Can you work these out from the model? Positions are in its coordinate system, mm. A direction names the side the tool comes from. Give positions to 0.01 mm unless a question says otherwise; leave off trailing zeros. Loops run counter-clockwise (first coordinate to the right, second up) from the corner with the lowest first, then second, coordinate; pieces in that order, holes last. Notation, with made-up numbers: (56.25, -17.5) -> (79.25, -17.5) arc R22 cw to (79.25, 13.5) -> close; hole circle Ø8 at (41.25, -32). An arc over 180 degrees is marked (long way). Return JSON: item names as keys, results as strings. Group by question number.
Q1. Suppose I cut it at A-A, the plane y = 155. Please give me the cut outline in (x, z) (1 decimal).
Q2. Thinking about a two-plate mould opening in X: for faces 1 (the flat face through (1, 47.625, 181)), 2 (the flat face through (-74.612, 143, 182)), 3 (the flat face through (-1, 143, 188.912)), which applies, pulls with the +X half, pulls with the -X half, needs draft (parallel to the pull), parting line crosses it, or undercut?
Q3. Will these pins go through, and if not, where does the flat tip stop? pin 1 (4 mm diameter, centred on x = 42, y = 159.5, fed in from -Z) (3 decimals); pin 2 (0.8 mm diameter, centred on x = -74, z = 180.5, fed in from +Y); pin 3 (4 mm diameter, centred on y = 71.44, z = 180.98, fed in from -X); pin 4 (3 mm diameter, centred on x = -55.5, z = 182, fed in from +Y) (3 decimals).
Q4. Suppose I cut it at B-B, the plane x = -1.5. Please give me the cut outline in (y, z) (1 decimal), and give its area (3 significant figures).
Q5. I need wall thicknesses on line 1 along X through (y, z) = (184.5, 179) (1 decimal); line 2 along Z through (x, y) = (53, 94.5) (1 decimal); line 3 along Y through (x, z) = (-11, 178) (1 decimal). Which ranges of each line are inside material? Lowest first, please. Write a range as [from, to].
Q6. Which directions (+Z, -Z, +X, -X, +Y, -Y) give clear straight access to the entire face, cutting with the end or side of a thin tool? Please do faces 4 (the flat face through (73.025, 137, 181)), 5 (the flat face through (-1, 46.038, 182)).
```python
from build123d import *

# Parameters (mm, degrees)
F3_DEPTH = 12.7
F5_DEPTH = 1.5875
F6_R     = 2.5527
F7_DEPTH = 149.226


with BuildPart() as f3:
    # F2 (on offset) → F3 (new body)
    with BuildSketch(Plane.XY.offset(187.325)):
        Polygon((-73.025, 47.625), (-73.025, 223.8375), (-74.6125, 223.8375), (-74.6125, 46.0375), (74.6125, 46.0375), (74.6125, 223.8375), (73.025, 223.8375), (73.025, 47.625), align=None)
    extrude(amount=-F3_DEPTH)

    # F4 (on face) → F5 (join)
    with BuildSketch(Plane.XY.offset(187.325)):
        Polygon((-74.6125, 46.0375), (74.6125, 46.0375), (74.6125, 223.8375), (74.6125, 236.5375), (-74.6125, 236.5375), (-74.6125, 223.8375), align=None)
    extrude(amount=F5_DEPTH)

    # F6 (on face) → F7 (cut, through all)
    with BuildSketch(Plane.YZ.offset(74.6125)):
        with Locations((71.4375, 180.975)):
            Circle(F6_R)
        with Locations((198.4375, 180.975)):
            Circle(F6_R)
    extrude(amount=-F7_DEPTH, mode=Mode.SUBTRACT)


solid = f3.part
```
Ans:
{
 "1": {"outline": "(-74.6, 174.6) -> (-73, 174.6) -> (-73, 187.3) -> (73, 187.3) -> (73, 174.6) -> (74.6, 174.6) -> (74.6, 188.9) -> (-74.6, 188.9) -> close"},
 "2": {"face 1": "undercut", "face 2": "pulls with the -X half", "face 3": "needs draft"},
 "3": {"pin 1": "stops at z = 187.325", "pin 2": "stops at y = 223.84", "pin 3": "passes through", "pin 4": "stops at y = 47.625"},
 "4": {"outline": "(46, 174.6) -> (47.6, 174.6) -> (47.6, 187.3) -> (236.5, 187.3) -> (236.5, 188.9) -> (46, 188.9) -> close", "area": "323 mm^2"},
 "5": {"line 1": "x = [-74.6, -73], [73, 74.6]", "line 2": "z = [187.3, 188.9]", "line 3": "y = [46, 47.6]"},
 "6": {"face 4": "-Z, +Y", "face 5": "+Z, -Z, +X, -X, -Y"}
}
